```python
from build123d import *

# Parameters (mm, degrees)
SKICA1_W                                          = 75
SKICA1_H                                          = 120
SKICA1_W_2                                        = 35
SKICA1_H_2                                        = 80
P_IDAT_VYSUNUT_M1_DEPTH                           = 2.5
SKICA2_W                                          = 75
SKICA2_H                                          = 120
SKICA2_W_2                                        = 70
SKICA2_H_2                                        = 115
P_IDAT_VYSUNUT_M2_DEPTH                           = 15
KU_ELOV_ZAHLOUBEN_PRO_M4_ROUBU_SE_2_COUNT         = 2
KU_ELOV_ZAHLOUBEN_PRO_M4_ROUBU_SE_2_PITCH         = 50
KU_ELOV_ZAHLOUBEN_PRO_M4_ROUBU_SE_3_COUNT         = 2
KU_ELOV_ZAHLOUBEN_PRO_M4_ROUBU_SE_3_PITCH         = 105
KU_ELOV_ZAHLOUBEN_PRO_M4_ROUBU_SE_4_COUNT         = 2
KU_ELOV_ZAHLOUBEN_PRO_M4_ROUBU_SE_4_PITCH         = 116.297033496
ODEBRAT_VYSUNUT_M4_DEPTH                          = 10
P_IDAT_VYSUNUT_M3_DEPTH                           = 7.5
SKICA22_W                                         = 70
SKICA22_H                                         = 2
P_IDAT_VYSUNUT_M4_DEPTH                           = 1.2
D_RY_PRO_KOL_K_VELIKOST_MM1_D                     = 3.8
D_RY_PRO_KOL_K_VELIKOST_MM1_DEPTH                 = 7.5
D_RY_PRO_KOL_K_VELIKOST_MM1_TIP                   = 1.141635176
SKICA27_W                                         = 2.5
SKICA27_H                                         = 10
P_IDAT_VYSUNUT_M5_DEPTH                           = 15
V_LCOV_ZAHLOUBEN_PRO_M3_ROUBY_S_K_NIC_D           = 3.4
V_LCOV_ZAHLOUBEN_PRO_M3_ROUBY_S_K_NIC_DEPTH       = 5
V_LCOV_ZAHLOUBEN_PRO_M3_ROUBY_S_K_NIC_CBORE_D     = 3.8
V_LCOV_ZAHLOUBEN_PRO_M3_ROUBY_S_K_NIC_CBORE_DEPTH = 4


with BuildPart() as part:
    # Skica1 → Přidat vysunutím1 (new body)
    with BuildSketch(Plane.XY):
        Rectangle(SKICA1_W, SKICA1_H)
        Rectangle(SKICA1_W_2, SKICA1_H_2, mode=Mode.SUBTRACT)
    extrude(amount=P_IDAT_VYSUNUT_M1_DEPTH)

    # Skica2 → Přidat vysunutím2 (add)
    with BuildSketch(Plane.XY.offset(2.5)):
        Rectangle(SKICA2_W, SKICA2_H)
        Rectangle(SKICA2_W_2, SKICA2_H_2, mode=Mode.SUBTRACT)
    extrude(amount=P_IDAT_VYSUNUT_M2_DEPTH)

    # Skica15 → Kuželové zahloubení pro M4 šroubu se zápustnou hlavou plochou2 (revolve, cut)
    with BuildSketch(Plane(origin=(25, 52.5, 2.5), x_dir=(0, -1, 0), z_dir=(1, 0, 0))):
        Polygon((0, 0), (0, 2.5), (2.25, 2.5), (2.25, 2.45), (4.7, 0), align=None)
    ku_elov_zahlouben_pro_m4_roubu_se_z_p = revolve(axis=Axis((25, 52.5, 8.85), (0, 0, -1)), mode=Mode.SUBTRACT)

    # Ku_elov_ zahlouben_ pro M4 _roubu se 2: Kuželové zahloubení pro M4 šroubu se zápustnou hlavou plochou2 ×2
    with Locations(*[(-i * KU_ELOV_ZAHLOUBEN_PRO_M4_ROUBU_SE_2_PITCH, 0, 0) for i in range(1, KU_ELOV_ZAHLOUBEN_PRO_M4_ROUBU_SE_2_COUNT)]):
        add(ku_elov_zahlouben_pro_m4_roubu_se_z_p, mode=Mode.SUBTRACT)

    # Ku_elov_ zahlouben_ pro M4 _roubu se 3: Kuželové zahloubení pro M4 šroubu se zápustnou hlavou plochou2 ×2
    with Locations(*[(0, -i * KU_ELOV_ZAHLOUBEN_PRO_M4_ROUBU_SE_3_PITCH, 0) for i in range(1, KU_ELOV_ZAHLOUBEN_PRO_M4_ROUBU_SE_3_COUNT)]):
        add(ku_elov_zahlouben_pro_m4_roubu_se_z_p, mode=Mode.SUBTRACT)

    # Ku_elov_ zahlouben_ pro M4 _roubu se 4: Kuželové zahloubení pro M4 šroubu se zápustnou hlavou plochou2 ×2
    with Locations(*[Vector(-0.42993358039234786, -0.9028605188239304, 0) * (i * KU_ELOV_ZAHLOUBEN_PRO_M4_ROUBU_SE_4_PITCH) for i in range(1, KU_ELOV_ZAHLOUBEN_PRO_M4_ROUBU_SE_4_COUNT)]):
        add(ku_elov_zahlouben_pro_m4_roubu_se_z_p, mode=Mode.SUBTRACT)

    # Skica20 → Odebrat vysunutím4 (cut)
    with BuildSketch(Plane.XZ.offset(60)):
        Polygon((0, 9.5), (-20, 9.5), (-20, 17.5), (20, 17.5), (20, 9.5), align=None)
    extrude(amount=-ODEBRAT_VYSUNUT_M4_DEPTH, mode=Mode.SUBTRACT)

    # Skica21 → Přidat vysunutím3 (add)
    with BuildSketch(Plane.XY.offset(2.5)):
        Polygon((35, -47.8), (-35, -47.8), (-35, 10.2), (-17.5, 10.2), (-17.5, -40), (17.5, -40), (17.5, 10.2), (35, 10.2), align=None)
    extrude(amount=P_IDAT_VYSUNUT_M3_DEPTH)

    # Skica22 → Přidat vysunutím4 (add)
    with BuildSketch(Plane.XY.offset(10)):
        with Locations((0, -46.8)):
            Rectangle(SKICA22_W, SKICA22_H)
    extrude(amount=P_IDAT_VYSUNUT_M4_DEPTH)

    # Díry pro kolík, velikost mm1
    with Locations(Plane.XY.offset(10)):
        with Locations((32, -17.8), (-32, -17.8)):
            Hole(D_RY_PRO_KOL_K_VELIKOST_MM1_D / 2, depth=D_RY_PRO_KOL_K_VELIKOST_MM1_DEPTH)
            with Locations((0, 0, -(D_RY_PRO_KOL_K_VELIKOST_MM1_DEPTH + D_RY_PRO_KOL_K_VELIKOST_MM1_TIP / 2))):  # 118° drill point
                Cone(0, D_RY_PRO_KOL_K_VELIKOST_MM1_D / 2, D_RY_PRO_KOL_K_VELIKOST_MM1_TIP, mode=Mode.SUBTRACT)

    # Skica27 → Přidat vysunutím5 (add)
    with BuildSketch(Plane.XY.offset(2.5)):
        with Locations((33.75, 37.5)):
            Rectangle(SKICA27_W, SKICA27_H)
        with Locations((-33.75, 37.5)):
            Rectangle(SKICA27_W, SKICA27_H)
    p_idat_vysunut_m5 = extrude(amount=P_IDAT_VYSUNUT_M5_DEPTH)

    # Zrcadlit1: Přidat vysunutím5 across plane
    add(p_idat_vysunut_m5.mirror(Plane.ZX))

    # Válcové zahloubení pro M3 šrouby s kónickou hlavou1
    with Locations(Plane(origin=(-32.5, 0, 0), x_dir=(0, 0, -1), z_dir=(1, 0, 0))):
        with Locations((-12.5, -37.5), (-12.5, 37.5)):
            v_lcov_zahlouben_pro_m3_rouby_s_k_nic = CounterBoreHole(V_LCOV_ZAHLOUBEN_PRO_M3_ROUBY_S_K_NIC_D / 2, V_LCOV_ZAHLOUBEN_PRO_M3_ROUBY_S_K_NIC_CBORE_D / 2, V_LCOV_ZAHLOUBEN_PRO_M3_ROUBY_S_K_NIC_CBORE_DEPTH, depth=V_LCOV_ZAHLOUBEN_PRO_M3_ROUBY_S_K_NIC_DEPTH)

    # Zrcadlit2: Válcové zahloubení pro M3 šrouby s kónickou hlavou1 across plane
    add(v_lcov_zahlouben_pro_m3_rouby_s_k_nic.mirror(Plane(origin=(0, 0, 0), x_dir=(0, 0, 1), z_dir=(1, 0, 0))), mode=Mode.SUBTRACT)


solid = part.part
```
Here's how the part is built. I have some questions about the finished solid (model axes, mm). A direction names the side the tool comes from. Give positions to 0.01 mm unless a question says otherwise; leave off trailing zeros. Write each loop counter-clockwise with the first axis right and the second up, starting at its lowest first coordinate (ties: lowest second). Pieces come first, ordered by that corner, then holes. Notation, with made-up numbers: M -17,41.25 L 22,41.25 A4 ccw 22,48.25 Z; hole C 3,72 d8. An arc over 180 degrees is marked long. Put each result on its own line as item: value. Start each with the question number.
Item 1: If we section it at A-A, the plane y = 16: Write out the boundary of the cut face in (x, z), then the cut area to 3 significant figures.
Item 2: Thinking about a two-plate mould opening in Y: for faces 1 (the flat face through (0, -53, 2.5)), 2 (the flat face through (-1, 60, 9)), 3 (the flat face through (24, 1, 0)), which applies, +Y half, -Y half, draft (parallel to the pull), parting line (faces both ways), or undercut?
Item 3: If we section it at B-B, the plane x = 5: Write out the boundary of the cut face in (y, z).
Item 4: Will these pins go through, and if not, where does the flat tip stop? pin 1 (5 mm diameter, centred on x = 2, y = 44, fed in from -Z); pin 2 (1.2 mm diameter, centred on x = 4.5, y = -58.5, fed in from +Z).
Item 5: I need wall thicknesses on L1, parallel to Y at x = 32, z = 5.5; L2, parallel to Y at x = -29, z = 5; L3, parallel to X at y = -37, z = 2.5. Which ranges of each line are inside material? Lowest first, please. Write a range as from..to.
Item 6: On a 3-axis mill with a long thin cutter (end or side, diameter ignored), from which of +Z, -Z, +X, -X, +Y, -Y can I reach the whole of each face in a straight line? I mean faces 4 (the flat face through (0, -59, 9.5)), 5 (the flat face through (0, 40, 1)), 6 (the cylindrical face through (-34.472, -39.186, 11.623)), 7 (the flat face through (32.5, -37, 15)). Say none if no direction works.
Item 7: If we section it at D-D, the plane y = -37.5: Write out the boundary of the cut face in (x, z), then the cut area to 3 significant figures.
Item 8: If we section it at C-C, the plane z = 7.75: Write out the boundary of the cut face in (x, y).
Values:
1. outline: M -37.5,0 L -17.5,0 L -17.5,2.5 L -35,2.5 L -35,17.5 L -37.5,17.5 Z; M 17.5,0 L 37.5,0 L 37.5,17.5 L 35,17.5 L 35,2.5 L 17.5,2.5 Z
1. area: 175 mm²
2. face 1: undercut
2. face 2: +Y half
2. face 3: draft
3. outline: M -60,0 L -40,0 L -40,10 L -45.8,10 L -45.8,11.2 L -47.8,11.2 L -47.8,2.5 L -57.5,2.5 L -57.5,9.5 L -60,9.5 Z; M 40,0 L 60,0 L 60,17.5 L 57.5,17.5 L 57.5,2.5 L 40,2.5 Z
4. pin 1: z = 0
4. pin 2: z = 9.5
5. L1: -60..-57.5, -47.8..-19.7, -15.9..10.2, 57.5..60
5. L2: -60..-57.5, -47.8..10.2, 57.5..60
5. L3: -37.5..-17.5, 17.5..37.5
6. face 4: +Z, -Y
6. face 5: +Z, -Z
6. face 6: none
6. face 7: +Z
7. outline: M -37.5,0 L -17.5,0 L -17.5,10 L -32.5,10 L -32.5,10.6 L -36.5,10.6 L -36.5,10.8 L -37.5,10.8 Z; M -37.5,14.2 L -36.5,14.2 L -36.5,14.4 L -32.5,14.4 L -32.5,17.5 L -37.5,17.5 Z; M 17.5,0 L 37.5,0 L 37.5,10.8 L 36.5,10.8 L 36.5,10.6 L 32.5,10.6 L 32.5,10 L 17.5,10 Z; M 32.5,14.4 L 36.5,14.4 L 36.5,14.2 L 37.5,14.2 L 37.5,17.5 L 32.5,17.5 Z
7. area: 438 mm²
8. outline: M -37.5,-60 L 37.5,-60 L 37.5,60 L -37.5,60 Z; hole M -35,-57.5 L 35,-57.5 L 35,-47.8 L -35,-47.8 Z; hole M -35,10.2 L -17.5,10.2 L -17.5,-40 L 17.5,-40 L 17.5,10.2 L 35,10.2 L 35,32.5 L 32.5,32.5 L 32.5,42.5 L 35,42.5 L 35,57.5 L -35,57.5 L -35,42.5 L -32.5,42.5 L -32.5,32.5 L -35,32.5 Z; hole C -32,-17.8 d3.8; hole C 32,-17.8 d3.8
